```python
from build123d import *

# Parameters (mm, degrees)
BOSS_EXTRUDE1_DEPTH              = 330.200001
BOSS_EXTRUDE1_DEPTH_BACK         = 330.200001
SKETCH3_W                        = 50.8
SKETCH3_H                        = 25.4
SKETCH3_W_2                      = 44.45
SKETCH3_H_2                      = 19.05
F_1_4_0_25_DIAMETER_HOLE3_D      = 6.35
F_1_4_0_25_DIAMETER_HOLE4_D      = 6.35
F_1_4_0_25_DIAMETER_HOLE5_D      = 6.35
F_1_4_0_25_DIAMETER_HOLE6_D      = 6.35
F_1_4_0_25_DIAMETER_HOLE7_D      = 6.35
F_1_4_0_25_DIAMETER_HOLE8_D      = 6.35
F_13_64_0_20313_DIAMETER_HOLE1_D = 5.159502
F_1_2_0_5_DIAMETER_HOLE1_D       = 12.7
F_1_2_0_5_DIAMETER_HOLE1_DEPTH   = 6.35
F_1_2_0_5_DIAMETER_HOLE1_TIP     = 3.815464931
F_10_CLEARANCE_HOLE4_AT_2_COUNT  = 2
F_10_CLEARANCE_HOLE4_AT_2_PITCH  = 26.422860684
F_10_CLEARANCE_HOLE4_AT_3_COUNT  = 2
F_10_CLEARANCE_HOLE4_AT_3_PITCH  = 32.162957462
F_10_CLEARANCE_HOLE4_AT_4_COUNT  = 2
F_10_CLEARANCE_HOLE4_AT_4_PITCH  = 33.11362798
SKETCH47_R                       = 14.2875
CUT_EXTRUDE1_DEPTH               = 333.148100492
TAP_DRILL_FOR_8_32_TAP1_D        = 3.4544
F_1_4_0_25_DIAMETER_HOLE9_D      = 6.35


with BuildPart() as part:
    # Sketch3 → Boss-Extrude1 (new, two sides: drawn at the far end of the back side and taken through both)
    with BuildSketch(Plane.XY.offset(-BOSS_EXTRUDE1_DEPTH_BACK)):
        Rectangle(SKETCH3_W, SKETCH3_H)
        Rectangle(SKETCH3_W_2, SKETCH3_H_2, mode=Mode.SUBTRACT)
    extrude(amount=BOSS_EXTRUDE1_DEPTH + BOSS_EXTRUDE1_DEPTH_BACK)

    # 1/4 (0.25) Diameter Hole3 (through all)
    with Locations(Plane.ZY.offset(25.4)):
        with Locations((-317.500000508, 0)):
            Hole(F_1_4_0_25_DIAMETER_HOLE3_D / 2)

    # 1/4 (0.25) Diameter Hole4 (through all)
    with Locations(Plane.ZY.offset(25.4)):
        with Locations((292.100000508, 0), (317.500000508, 0)):
            Hole(F_1_4_0_25_DIAMETER_HOLE4_D / 2)

    # 1/4 (0.25) Diameter Hole5 (through all)
    with Locations(Plane(origin=(25.4, 0, 0), x_dir=(0, 0, -1), z_dir=(1, 0, 0))):
        with Locations((292.100000508, 0), (266.700000508, 0)):
            Hole(F_1_4_0_25_DIAMETER_HOLE5_D / 2)

    # 1/4 (0.25) Diameter Hole6 (through all)
    with Locations(Plane(origin=(25.4, 0, 0), x_dir=(0, 0, -1), z_dir=(1, 0, 0))):
        with Locations((215.900000508, 0), (241.300000508, 0)):
            Hole(F_1_4_0_25_DIAMETER_HOLE6_D / 2)

    # 1/4 (0.25) Diameter Hole7 (through all)
    with Locations(Plane(origin=(25.4, 0, 0), x_dir=(0, 0, -1), z_dir=(1, 0, 0))):
        with Locations((-190.5, 0), (-215.9, 0)):
            Hole(F_1_4_0_25_DIAMETER_HOLE7_D / 2)

    # 1/4 (0.25) Diameter Hole8 (through all)
    with Locations(Plane(origin=(25.4, 0, 0), x_dir=(0, 0, -1), z_dir=(1, 0, 0))):
        with Locations((-266.7, 0), (-241.3, 0)):
            Hole(F_1_4_0_25_DIAMETER_HOLE8_D / 2)

    # 13/64 (0.20313) Diameter Hole1 (through all)
    with Locations(Plane(origin=(25.4, 0, 0), x_dir=(0, 0, -1), z_dir=(1, 0, 0))):
        with Locations((-152.4, 0), (177.8, 0)):
            Hole(F_13_64_0_20313_DIAMETER_HOLE1_D / 2)

    # 1/2 (0.5) Diameter Hole1
    with Locations(Plane.ZY.offset(25.4)):
        with Locations((-128.5875, 1.016e-06), (-103.1875, 1.016e-06), (77.7875, 1.016e-06), (103.1875, 1.016e-06)):
            Hole(F_1_2_0_5_DIAMETER_HOLE1_D / 2, depth=F_1_2_0_5_DIAMETER_HOLE1_DEPTH)
            with Locations((0, 0, -(F_1_2_0_5_DIAMETER_HOLE1_DEPTH + F_1_2_0_5_DIAMETER_HOLE1_TIP / 2))):  # 118° drill point
                Cone(0, F_1_2_0_5_DIAMETER_HOLE1_D / 2, F_1_2_0_5_DIAMETER_HOLE1_TIP, mode=Mode.SUBTRACT)

    # Sketch46 → #10 Clearance Hole4 (revolve, cut)
    with BuildSketch(Plane(origin=(13.81901292, -12.7, 101.782101571), x_dir=(0, 0, -1), z_dir=(1, 0, 0))):
        Polygon((0, 0), (0, 25.4), (5.2197, 25.4), (2.4892, 22.258919064), (2.4892, 0), align=None)
    f_10_clearance_hole4 = revolve(axis=Axis((13.81901292, -19.05, 101.782101571), (0, 1, 0)), mode=Mode.SUBTRACT)

    # #10 Clearance Hole4 at 2: #10 Clearance Hole4 ×2
    with Locations(*[Vector(0.15562183859411732, 0, 0.9878167053419306) * (i * F_10_CLEARANCE_HOLE4_AT_2_PITCH) for i in range(1, F_10_CLEARANCE_HOLE4_AT_2_COUNT)]):
        add(f_10_clearance_hole4, mode=Mode.SUBTRACT)

    # #10 Clearance Hole4 at 3: #10 Clearance Hole4 ×2
    with Locations(*[Vector(-0.8593123276123449, 0, 0.511451193774591) * (i * F_10_CLEARANCE_HOLE4_AT_3_PITCH) for i in range(1, F_10_CLEARANCE_HOLE4_AT_3_COUNT)]):
        add(f_10_clearance_hole4, mode=Mode.SUBTRACT)

    # #10 Clearance Hole4 at 4: #10 Clearance Hole4 ×2
    with Locations(*[Vector(-0.9588197348681927, 0, -0.284015344703924) * (i * F_10_CLEARANCE_HOLE4_AT_4_PITCH) for i in range(1, F_10_CLEARANCE_HOLE4_AT_4_COUNT)]):
        add(f_10_clearance_hole4, mode=Mode.SUBTRACT)

    # Sketch47 → Cut-Extrude1 (cut, through all)
    with BuildSketch(Plane.XZ.offset(12.7)):
        with Locations((-7.9375, 160.637603217)):
            Circle(SKETCH47_R)
    extrude(amount=-CUT_EXTRUDE1_DEPTH, mode=Mode.SUBTRACT)

    # Tap Drill for #8-32 Tap1 (through all)
    with Locations(Plane(origin=(0, -12.7, 0), x_dir=(-1, 0, 0), z_dir=(0, -1, 0))):
        with Locations((-4.814463692, -173.389566909)):
            Hole(TAP_DRILL_FOR_8_32_TAP1_D / 2)

    # 1/4 (0.25) Diameter Hole9 (through all)
    with Locations(Plane(origin=(0, -12.7, 0), x_dir=(-1, 0, 0), z_dir=(0, -1, 0))):
        with Locations((-15.875, 187.325)):
            Hole(F_1_4_0_25_DIAMETER_HOLE9_D / 2)


solid = part.part
```
Verification items for the finished model (mm, model axes). A direction names the side the tool comes from. Give positions to 0.01 mm unless a question says otherwise; leave off trailing zeros. Order: outer loops, then holes, each group sorted by start corner. A loop starts at its lowest first (then second) coordinate and runs counter-clockwise, first axis right, second up. Notation, with made-up numbers: M 60,34 L 82,34 A31 cw 82,64 Z; hole C 60,57.5 d11. An arc over 180 degrees is marked long. Return JSON: item names as keys, results as strings. Group by question number.
1) Section check B-B on x = -3. Record the cut outline in (y, z) (3 decimals), and give its area (3 significant figures).
2) Mould release check, pull along X, two halves, no side actions. Record for faces 1 (the face through (-23.79, 0.279, -122.244)), 2 (the face through (-9.797, 11.09, 174.804)), 3 (the face through (-25.4, 0, -5)): pulls with the +X half, pulls with the -X half, needs draft (parallel to the pull), parting line crosses it, or undercut.
3) Section check A-A on z = -162. Record the cut outline in (x, y) (3 decimals), and give its area (3 significant figures).
4) Scan lines: line 1 (Y direction, x = 7, z = -41) (3 decimals); line 2 (X direction, y = 6.25, z = 222) (3 decimals); line 3 (Y direction, x = -23, z = 215). Record each from-to range of solid material in increasing order.
5) Go/stop test with a flat-tipped pin: pin 1 Ø4 at (y, z) = (0, -177.8) entering from +X. Record where the tip stops, or that it passes through.
6) Access from +Z, -Z, +X, -X, +Y, -Y to the whole of each face (thin tool, end or side, straight path). Record for faces 4 (the face through (-18.72, 9.71, 89.88)), 5 (the face through (0, -9.525, -5)), 6 (the face through (-23.79, 1.91, 97.13)).
Answer block:
{
 "1": {"outline": "M -12.7,-330.2 L -9.525,-330.2 L -9.525,147.23 L -12.7,147.23 Z; M -12.7,174.045 L -9.525,174.045 L -9.525,330.2 L -12.7,330.2 Z; M 9.525,-330.2 L 12.7,-330.2 L 12.7,147.23 L 9.525,147.23 Z; M 9.525,174.045 L 12.7,174.045 L 12.7,330.2 L 9.525,330.2 Z", "area": "4,020 mm^2"},
 "2": {"face 1": "needs draft", "face 2": "undercut", "face 3": "pulls with the -X half"},
 "3": {"outline": "M -25.4,-12.7 L 25.4,-12.7 L 25.4,12.7 L -25.4,12.7 Z; hole M -22.225,-9.525 L 22.225,-9.525 L 22.225,9.525 L -22.225,9.525 Z", "area": "444 mm^2"},
 "4": {"line 1": "y = -12.7 to -9.525, 9.525 to 12.7", "line 2": "x = -25.4 to -22.225, 22.225 to 25.4", "line 3": "y = -12.7 to -3.04, 3.04 to 12.7"},
 "5": {"pin 1": "passes through"},
 "6": {"face 4": "+Y", "face 5": "+Z, -Z", "face 6": "-X"}
}
